from build123d import *

# Parameters (mm, degrees)
SKETCH1_W           = 3.175
SKETCH1_H           = 12.7
SKETCH3_R           = 67.061060388
SKETCH3_R_2         = 66.267310388
BOSS_EXTRUDE1_DEPTH = 12.7
FILLET2_R           = 0.79375


with BuildPart() as part:
    # Sketch1 → Revolve3 (revolve)
    with BuildSketch(Plane.XY):
        with BuildLine():
            Line((69.85, 0), (69.85, 76.2))
            ThreePointArc((69.85, 76.2), (49.391408666, 125.591408666), (0, 146.05))
            Line((0, 146.05), (0, 139.7))
            ThreePointArc((0, 139.7), (44.901280605, 121.101280605), (63.5, 76.2))
            Line((63.5, 76.2), (63.5, 0))
            Line((63.5, 0), (69.85, 0))
        make_face()
        with Locations((68.2625, -6.35)):
            Rectangle(SKETCH1_W, SKETCH1_H)
    revolve(axis=Axis((0, 146.05, 0), (0, -1, 0)))

    # Sketch3 → Boss-Extrude1 (add)
    with BuildSketch(Plane(origin=(0, 0, 0), x_dir=(-1, 0, 0), z_dir=(0, -1, 0))):
        Circle(SKETCH3_R)
        Circle(SKETCH3_R_2, mode=Mode.SUBTRACT)
    extrude(amount=BOSS_EXTRUDE1_DEPTH)

    # Fillet2
    fillet2_edges = [part.edges().sort_by_distance(p)[0] for p in [
        (66.267310388, -12.7, 0),
    ]]
    fillet(fillet2_edges, radius=FILLET2_R)


solid = part.part
Could you check a few things on this model? Use its own coordinates, in mm. Give positions to 0.01 mm unless a question says otherwise; leave off trailing zeros. Write each loop counter-clockwise with the first axis right and the second up, starting at its lowest first coordinate (ties: lowest second). Pieces come first, ordered by that corner, then holes. Notation, with made-up numbers: (-21.75, 53.5) -> (4.25, 53.5) arc R16 ccw to (4.25, 76.5) -> close; hole circle Ø2 at (84.25, -34). An arc over 180 degrees is marked (long way). Answer as a JSON object with one key per item and string values.
Q1. Suppose I cut it at A-A on z = 0. Write out the boundary of the cut face in (x, y), then the cut area to 3 significant figures.
Taken from the geometry:
{"outline": "(-69.85, -12.7) -> (-67.06, -12.7) arc R0.79 ccw to (-66.27, -11.91) -> (-66.27, 0) -> (-63.5, 0) -> (-63.5, 76.2) arc R63.5 cw to (63.5, 76.2) -> (63.5, 0) -> (66.27, 0) -> (66.27, -11.91) arc R0.79 ccw to (67.06, -12.7) -> (69.85, -12.7) -> (69.85, 76.2) arc R69.85 ccw to (-69.85, 76.2) -> close", "area": "2,390 mm²"}
Q2. Suppose I cut it at B-B on x = 0. Write out the boundary of the cut face in (y, z), then the cut area to 3 significant figures.
Taken from the geometry:
{"outline": "(-12.7, -69.85) -> (76.2, -69.85) arc R69.85 ccw to (76.2, 69.85) -> (-12.7, 69.85) -> (-12.7, 67.06) arc R0.79 ccw to (-11.91, 66.27) -> (0, 66.27) -> (0, 63.5) -> (76.2, 63.5) arc R63.5 cw to (76.2, -63.5) -> (0, -63.5) -> (0, -66.27) -> (-11.91, -66.27) arc R0.79 ccw to (-12.7, -67.06) -> close", "area": "2,390 mm²"}
Q3. Suppose I cut it at C-C on y = 131.5. Write out the boundary of the cut face in (x, z), then the cut area to 3 significant figures.
Taken from the geometry:
{"outline": "circle Ø85.34 at (0, 0); hole circle Ø62.42 at (0, 0)", "area": "2,660 mm²"}
Q4. We'd pull the mould along X, two halves only. Please class faces 1 (the cylindrical face through (-13.77, 37.57, -61.99)), 2 (the cylindrical face through (-55.431, 32.372, -42.503)), 3 (the flat face through (26, -12.7, 62)): released by +X, released by -X, zero draft, split by the parting line, or undercut.
Taken from the geometry:
{"face 1": "undercut", "face 2": "split by the parting line", "face 3": "zero draft"}
Q5. Please list where these lines run through material, in increasing order: L1, parallel to X at y = 71, z = 1.5; L2, parallel to Z at x = 0, y = 40.5; L3, parallel to Z at x = 0, y = -6.
Taken from the geometry:
{"L1": "x = -69.83 to -63.48, 63.48 to 69.83", "L2": "z = -69.85 to -63.5, 63.5 to 69.85", "L3": "z = -69.85 to -66.27, 66.27 to 69.85"}
Q6. Will these pins go through, and if not, where does the flat tip stop? pin 1 Ø8 at (x, y) = (-17, 64.5) entering from -Z; pin 2 Ø6 at (y, z) = (22.5, -31.5) entering from -X; pin 3 Ø10 at (x, y) = (-39, 93) entering from +Z.
Taken from the geometry:
{"pin 1": "stops at z = -68.63", "pin 2": "stops at x = -63.77", "pin 3": "stops at z = 58.95"}
